CAD build for the part. Positions are in the model's coordinates, mm. A direction names the side the tool comes from. Coordinates: 2 decimals unless noted, no trailing zeros. Order: outer loops, then holes, each group sorted by start corner. A loop starts at its lowest first (then second) coordinate and runs counter-clockwise, first axis right, second up. Notation, with made-up numbers: M 40,-6.5 L 92,-6.5 A21 cw 92,14.5 Z; hole C 71,-24.75 d8. An arc over 180 degrees is marked long. Write item = value, one per line.
from build123d import *

# Parameters (mm, degrees)
SKETCH1_W           = 76.4
SKETCH1_H           = 56.4
SKETCH1_R           = 19.5
SKETCH1_R_2         = 3
BOSS_EXTRUDE1_DEPTH = 6
SKETCH2_W           = 9.5
SKETCH2_H           = 56.4
BOSS_EXTRUDE2_DEPTH = 40
FILLET1_R           = 3
SKETCH3_W           = 40
SKETCH3_H           = 8
BOSS_EXTRUDE3_DEPTH = 12
SKETCH4_W           = 40
SKETCH4_H           = 8
BOSS_EXTRUDE4_DEPTH = 12
FILLET2_R           = 4
SKETCH5_R           = 3
CUT_EXTRUDE1_DEPTH  = 12
CHAMFER1_SIZE       = 40


with BuildPart() as part:
    # Sketch1 → Boss-Extrude1 (new body)
    with BuildSketch(Plane.XY):
        with Locations((38.2, 28.2)):
            Rectangle(SKETCH1_W, SKETCH1_H)
        with Locations((38.2, 28.2)):
            Circle(SKETCH1_R, mode=Mode.SUBTRACT)
        with Locations((14.63, 51.77)):
            Circle(SKETCH1_R_2, mode=Mode.SUBTRACT)
        with Locations((61.77, 51.77)):
            Circle(SKETCH1_R_2, mode=Mode.SUBTRACT)
        with Locations((61.77, 4.63)):
            Circle(SKETCH1_R_2, mode=Mode.SUBTRACT)
        with Locations((14.63, 4.63)):
            Circle(SKETCH1_R_2, mode=Mode.SUBTRACT)
    extrude(amount=BOSS_EXTRUDE1_DEPTH)

    # Sketch2 → Boss-Extrude2 (add)
    with BuildSketch(Plane(origin=(0, 0, 0), x_dir=(-1, 0, 0), z_dir=(0, 0, -1))):
        with Locations((-71.65, 28.2)):
            Rectangle(SKETCH2_W, SKETCH2_H)
        with Locations((-4.75, 28.2)):
            Rectangle(SKETCH2_W, SKETCH2_H)
    extrude(amount=BOSS_EXTRUDE2_DEPTH)

    # Fillet1
    fillet1_edges = [part.edges().sort_by_distance(p)[0] for p in [
        (76.4, 28.2, 6),
        (0, 28.2, 6),
    ]]
    fillet(fillet1_edges, radius=FILLET1_R)

    # Sketch3 → Boss-Extrude3 (add)
    with BuildSketch(Plane.ZY):
        with Locations((-20, 4)):
            Rectangle(SKETCH3_W, SKETCH3_H)
    extrude(amount=BOSS_EXTRUDE3_DEPTH)

    # Sketch4 → Boss-Extrude4 (add)
    with BuildSketch(Plane(origin=(76.4, 0, 0), x_dir=(0, 0, -1), z_dir=(1, 0, 0))):
        with Locations((20, 4)):
            Rectangle(SKETCH4_W, SKETCH4_H)
    extrude(amount=BOSS_EXTRUDE4_DEPTH)

    # Fillet2
    fillet2_edges = [part.edges().sort_by_distance(p)[0] for p in [
        (-12, 4, -40),
        (-12, 4, 0),
        (88.4, 4, 0),
        (88.4, 4, -40),
    ]]
    fillet(fillet2_edges, radius=FILLET2_R)

    # Sketch5 → Cut-Extrude1 (cut)
    with BuildSketch(Plane(origin=(0, 8, 0), x_dir=(1, 0, 0), z_dir=(0, 1, 0))):
        with Locations(Location((-6, 32, 0), (0, 0, 270))):
            Circle(SKETCH5_R)
        with Locations(Location((-6, 8, 0), (0, 0, 270))):
            Circle(SKETCH5_R)
        with Locations(Location((82.4, 32, 0), (0, 0, 270))):
            Circle(SKETCH5_R)
        with Locations(Location((82.4, 8, 0), (0, 0, 270))):
            Circle(SKETCH5_R)
    extrude(amount=-CUT_EXTRUDE1_DEPTH, mode=Mode.SUBTRACT)

    # Chamfer1
    chamfer1_edges = [part.edges().sort_by_distance(p)[0] for p in [
        (4.75, 56.4, -40),
        (71.65, 56.4, -40),
    ]]
    chamfer(chamfer1_edges, length=CHAMFER1_SIZE)


solid = part.part
(1) Slice it at B-B, the plane y = 28.2. Write the cut outline in (x, z).
Evaluation:
outline = M 0,-28.2 L 9.5,-28.2 L 9.5,0 L 18.7,0 L 18.7,6 L 3,6 A3 ccw 0,3 Z; M 57.7,0 L 66.9,0 L 66.9,-28.2 L 76.4,-28.2 L 76.4,3 A3 ccw 73.4,6 L 57.7,6 Z
(2) Pin check, flat tips, straight feed: pin 1 Ø12 at (y, z) = (40, -7) entering from -X; pin 2 Ø1 at (y, z) = (21.5, -31) entering from +X; pin 3 Ø9.5 at (x, y) = (14.63, 4.63) entering from -Z; pin 4 Ø5 at (x, z) = (-6, -32) entering from -Y. Stop position of each tip, or through.
Evaluation:
pin_1 = 0
pin_2 = 76.4
pin_3 = 0
pin_4 = through
(3) Slice it at C-C, the plane x = 38.2. Write the cut outline in (y, z), then the cut area to 3 significant figures.
Evaluation:
outline = M 0,0 L 8.7,0 L 8.7,6 L 0,6 Z; M 47.7,0 L 56.4,0 L 56.4,6 L 47.7,6 Z
area = 104 mm²
(4) Slice it at A-A, the plane x = -6. Write the cut outline in (y, z), then the cut area to 3 significant figures.
Evaluation:
outline = M 0,-40 L 8,-40 L 8,-35 L 0,-35 Z; M 0,-29 L 8,-29 L 8,-11 L 0,-11 Z; M 0,-5 L 8,-5 L 8,0 L 0,0 Z
area = 224 mm²
(5) Tool access for faces 1 (the face through (9.5, 22, -15)), 2 (the face through (80, 4, 0)), 3 (the face through (-6, 8, -20)), 4 (the face through (82, 8, -20)), 5 (the face through (71.7, 36.7, -19.7)): list every direction of +Z, -Z, +X, -X, +Y, -Y with a clear straight run to the whole face (end or side of a thin tool).
Evaluation:
face_1 = -Z, +Y, -Y
face_2 = +Z, +X, +Y, -Y
face_3 = +Z, -Z, -X, +Y
face_4 = +Z, -Z, +X, +Y
face_5 = -Z, +X, -X, +Y
(6) Pull direction X, two halves, no side cores. Call faces 6 (the face through (22, 41, 6)), 7 (the face through (87.197, 4.056, -1.141)), 8 (the face through (63.38, 54.3, 2.96)): +X half, -X half, draft (parallel to the pull), parting line (faces both ways), or undercut.
Evaluation:
face_6 = draft
face_7 = +X half
face_8 = undercut
(7) Slice it at D-D, the plane y = 4.63. State how many separate pieces and enclosed holes the cut face has, then the cut area to 3 significant figures.
Evaluation:
separate_pieces = 3
enclosed_holes = 4
area = 1,980 mm²
(8) Wall check: line 1 (Y direction, x = 61, z = 3); line 2 (X direction, y = 6, z = 2.5); line 3 (X direction, y = 17, z = -11). Give the ranges that are in metal, low to high. Write a range as from..to.
Evaluation:
line_1 = 0..1.73, 7.53..48.87, 54.67..56.4
line_2 = 0..11.96, 17.3..59.1, 64.44..76.4
line_3 = 0..9.5, 66.9..76.4
